Design review of the part built by this model. Coordinates are the model's own, in mm. Coordinates: 2 decimals unless noted, no trailing zeros. Loops run counter-clockwise (first coordinate to the right, second up) from the corner with the lowest first, then second, coordinate; pieces in that order, holes last. Notation, with made-up numbers: (47, 51) -> (53, 51) arc R14 ccw to (53, 69) -> close; hole circle Ø4 at (-30.5, -23). An arc over 180 degrees is marked (long way). Answer as a JSON object with one key per item and string values.
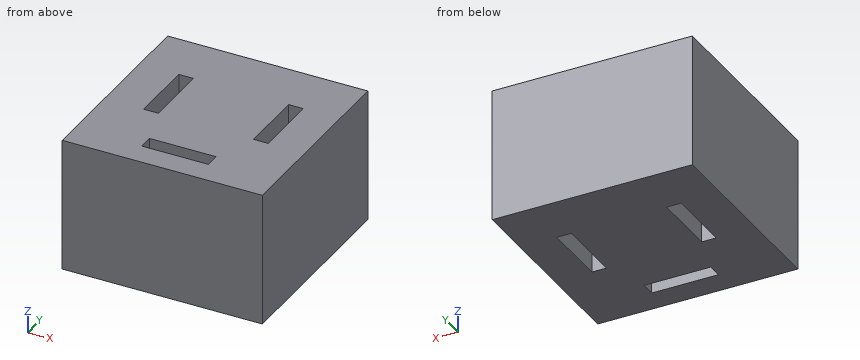
```python
from build123d import *

# Parameters (mm, degrees)
F0_W     = 38.1
F0_H     = 38.1
F0_W_2   = 12.7
F0_H_2   = 2.794
F0_W_3   = 2.794
F0_H_3   = 12.7
F1_DEPTH = 25.4
F2_DEPTH = 25.4


with BuildPart() as f1:
    # F0 (on Top) → F1 (new body)
    with BuildSketch(Plane.XY):
        Rectangle(F0_W, F0_H)
        with Locations((0, -13.044956)):
            Rectangle(F0_W_2, F0_H_2, mode=Mode.SUBTRACT)
        with Locations((-10.21277, 2.598171)):
            Rectangle(F0_W_3, F0_H_3, mode=Mode.SUBTRACT)
        with Locations((10.70081, 2.598171)):
            Rectangle(F0_W_3, F0_H_3, mode=Mode.SUBTRACT)
    extrude(amount=F1_DEPTH)

    # F0 (on Top) → F2 (cut)
    with BuildSketch(Plane.XY):
        Rectangle(F0_W, F0_H)
        with Locations((0, -13.044956)):
            Rectangle(F0_W_2, F0_H_2, mode=Mode.SUBTRACT)
        with Locations((-10.21277, 2.598171)):
            Rectangle(F0_W_3, F0_H_3, mode=Mode.SUBTRACT)
        with Locations((10.70081, 2.598171)):
            Rectangle(F0_W_3, F0_H_3, mode=Mode.SUBTRACT)
    extrude(amount=-F2_DEPTH, mode=Mode.SUBTRACT)


solid = f1.part
```
1) Add section C-C, the plane x = -4.5. Give the boundary of the cut face in (y, z), and give its area (3 significant figures).
Completed:
{"outline": "(-19.05, 0) -> (-14.44, 0) -> (-14.44, 25.4) -> (-19.05, 25.4) -> close; (-11.65, 0) -> (19.05, 0) -> (19.05, 25.4) -> (-11.65, 25.4) -> close", "area": "897 mm²"}
2) Add section B-B, the plane z = 8.25. Give the boundary of the cut face in (x, y), and give its area (3 significant figures).
Completed:
{"outline": "(-19.05, -19.05) -> (19.05, -19.05) -> (19.05, 19.05) -> (-19.05, 19.05) -> close; hole (-11.61, -3.75) -> (-8.82, -3.75) -> (-8.82, 8.95) -> (-11.61, 8.95) -> close; hole (-6.35, -14.44) -> (6.35, -14.44) -> (6.35, -11.65) -> (-6.35, -11.65) -> close; hole (9.3, -3.75) -> (12.1, -3.75) -> (12.1, 8.95) -> (9.3, 8.95) -> close", "area": "1,350 mm²"}
3) Wall thickness on probe 1 along X at (y, z) = (6, 17.75); probe 2 along Y at (x, z) = (11, 22.5); probe 3 along Y at (x, z) = (0, 14.25): over which ranges is each line inside the solid? List them lowest first.
Completed:
{"probe 1": "-19.05 to -11.61, -8.82 to 9.3, 12.1 to 19.05", "probe 2": "-19.05 to -3.75, 8.95 to 19.05", "probe 3": "-19.05 to -14.44, -11.65 to 19.05"}
4) Add section A-A, the plane y = 7.5. Give the boundary of the cut face in (x, z).
Completed:
{"outline": "(-19.05, 0) -> (-11.61, 0) -> (-11.61, 25.4) -> (-19.05, 25.4) -> close; (-8.82, 0) -> (9.3, 0) -> (9.3, 25.4) -> (-8.82, 25.4) -> close; (12.1, 0) -> (19.05, 0) -> (19.05, 25.4) -> (12.1, 25.4) -> close"}
